Geometry: final body of the model. Coordinates: model frame, mm. A direction names the side the tool comes from. Coordinates: 2 decimals unless noted, no trailing zeros. Loops run counter-clockwise (first coordinate to the right, second up) from the corner with the lowest first, then second, coordinate; pieces in that order, holes last. Notation, with made-up numbers: (11.5, 23) - (69.5, 23) arc R17 cw to (69.5, 46) - close; hole circle Ø6 at (82.5, 44.5). An arc over 180 degrees is marked (long way). Answer in a Markdown table with one row per item.
from build123d import *

# Parameters (mm, degrees)
F1_DEPTH = 5.08
F2_W     = 19.05
F2_H     = 12.7
F3_DEPTH = 50.8
F5_DEPTH = 19.05
F7_DEPTH = 19.05
F9_DEPTH = 5.08


with BuildPart() as f1:
    # F0 (on Top) → F1 (new body)
    with BuildSketch(Plane.XY):
        Polygon((0, 12.7), (0, 0), (19.05, 0), (76.2, 0), (76.2, 50.8), (0, 50.8), align=None)
    extrude(amount=F1_DEPTH)

    # F2 (on face) → F3 (join)
    with BuildSketch(Plane.XY.offset(5.08)):
        with Locations((9.525, 6.35)):
            Rectangle(F2_W, F2_H)
        with Locations((66.675, 6.35)):
            Rectangle(F2_W, F2_H)
    extrude(amount=F3_DEPTH)

    # F4 (on face) → F5 (join)
    with BuildSketch(Plane(origin=(0, 0, 0), x_dir=(0, -1, 0), z_dir=(-1, 0, 0))):
        with BuildLine():
            Line((-12.7, 55.88), (0, 55.88))
            ThreePointArc((0, 55.88), (-6.35, 62.23), (-12.7, 55.88))
        make_face()
        with BuildLine():
            ThreePointArc((-12.7, 55.88), (-6.35, 49.53), (0, 55.88))
            Line((0, 55.88), (-12.7, 55.88))
        make_face()
    extrude(amount=-F5_DEPTH)

    # F6 (on face) → F7 (join)
    with BuildSketch(Plane.YZ.offset(76.2)):
        with BuildLine():
            ThreePointArc((0, 55.88), (6.35, 49.53), (12.7, 55.88))
            Line((12.7, 55.88), (0, 55.88))
        make_face()
        with BuildLine():
            Line((0, 55.88), (12.7, 55.88))
            ThreePointArc((12.7, 55.88), (6.35, 62.23), (0, 55.88))
        make_face()
    extrude(amount=-F7_DEPTH)

    # F8 (on face) → F9 (cut)
    with BuildSketch(Plane.XY.offset(5.08)):
        with BuildLine():
            ThreePointArc((30.48, 25.4), (26.760256, 16.419744), (17.78, 12.7))
            Line((17.78, 12.7), (19.05, 12.7))
            Line((19.05, 12.7), (19.05, 0))
            Line((19.05, 0), (57.15, 0))
            Line((57.15, 0), (57.15, 12.7))
            Line((57.15, 12.7), (58.42, 12.7))
            ThreePointArc((58.42, 12.7), (49.439744, 16.419744), (45.72, 25.4))
            Line((45.72, 25.4), (45.72, 35.052))
            Line((45.72, 35.052), (30.48, 35.052))
            Line((30.48, 35.052), (30.48, 25.4))
        make_face()
    extrude(amount=-F9_DEPTH, mode=Mode.SUBTRACT)


solid = f1.part
(1) Ray query, probe 1 along X at (y, z) = (11, 45); probe 2 along Z at (x, y) = (45, 49); probe 3 along Y at (x, z) = (6.5, 33). Return the intervals inside material, ascending.
Verdict:
| item | result |
|---|---|
| probe 1 | x = 0 to 19.05, 57.15 to 76.2 |
| probe 2 | z = 0 to 5.08 |
| probe 3 | y = 0 to 12.7 |
(2) Cut plane C-C on x = 70.5. Output: boundary loops of the cut face in (y, z), then the cut area to 3 significant figures.
Verdict:
| item | result |
|---|---|
| outline | (0, 0) - (50.8, 0) - (50.8, 5.08) - (12.7, 5.08) - (12.7, 55.88) arc R6.35 ccw to (0, 55.88) - close |
| area | 967 mm² |
(3) First-contact query: pin 1 Ø15 at (x, z) = (9.5, 14.5) entering from +Y; pin 2 Ø12 at (x, y) = (33, 15.5) entering from +Z; pin 3 Ø2 at (x, y) = (57, 10.5) entering from +Z. Flat tips, straight axial feed; report the tip coordinate or a pass-through.
Verdict:
| item | result |
|---|---|
| pin 1 | stops at y = 12.7 |
| pin 2 | stops at z = 5.08 |
| pin 3 | stops at z = 61.39 |
(4) Cut plane D-D on y = 46.5. Output: boundary loops of the cut face in (x, z).
Verdict:
| item | result |
|---|---|
| outline | (0, 0) - (76.2, 0) - (76.2, 5.08) - (0, 5.08) - close |
(5) Pull-direction query (X, two-part tool) for faces 3 (the face through (45.72, 30, 3)), 4 (the face through (0, 10, 26)), 5 (the face through (38, 36, 5.08)); classes: pulls with the +X half, pulls with the -X half, needs draft (parallel to the pull), parting line crosses it, or undercut.
Verdict:
| item | result |
|---|---|
| face 3 | undercut |
| face 4 | pulls with the -X half |
| face 5 | needs draft |
(6) Access query for faces 1 (the face through (30.48, 30, 3)), 2 (the face through (9.39, 6.21, 62.23)). Directions: +Z, -Z, +X, -X, +Y, -Y. A direction counts if a zero-diameter tool reaches every point of the face in a straight line with its end or side. Return the directions, or none.
Verdict:
| item | result |
|---|---|
| face 1 | +Z, -Z, -Y |
| face 2 | +Z, +X, -X |
(7) Cut plane B-B on y = 6.35. Output: boundary loops of the cut face in (x, z), then the cut area to 3 significant figures.
Verdict:
| item | result |
|---|---|
| outline | (0, 0) - (19.05, 0) - (19.05, 62.23) - (0, 62.23) - close; (57.15, 0) - (76.2, 0) - (76.2, 62.23) - (57.15, 62.23) - close |
| area | 2,370 mm² |
(8) Cut plane A-A on z = 11.5. Output: boundary loops of the cut face in (x, y), then the cut area to 3 significant figures.
Verdict:
| item | result |
|---|---|
| outline | (0, 0) - (19.05, 0) - (19.05, 12.7) - (0, 12.7) - close; (57.15, 0) - (76.2, 0) - (76.2, 12.7) - (57.15, 12.7) - close |
| area | 484 mm² |
